The model under review builds one solid part; all positions refer to its coordinate system, in mm. A direction names the side the tool comes from. Give positions to 0.01 mm unless a question says otherwise; leave off trailing zeros. Write each loop counter-clockwise with the first axis right and the second up, starting at its lowest first coordinate (ties: lowest second). Pieces come first, ordered by that corner, then holes. Notation, with made-up numbers: M -6.75,28 L 51.25,28 A24 ccw 51.25,40 Z; hole C 32,25.25 d4. An arc over 180 degrees is marked long. Write each question's results on one line, items separated by ' | '. Start each with the question number.
from build123d import *

# Parameters (mm, degrees)
F0_R         = 4.7625
F0_R_2       = 1.5
F0_R_3       = 11.2530001
F1_DEPTH     = 3.175
F2_T1_DEPTH  = 34.0506804732
F2_T6_DEPTH  = 34.0506804732
F2_T11_DEPTH = 34.0506804732


# Not quite as in the source:
# - a fillet or chamfer that OpenCascade refuses, or shapes differently, is made with other operations: its cross-section is extruded or revolved along the edge and cut away or added


with BuildPart() as f1:
    # F0 (on Top) → F1 (new body)
    with BuildSketch(Plane.XY):
        with BuildLine():
            Line((15.875, 0), (12.7, 0))
            ThreePointArc((12.7, 0), (0, -12.7), (-12.7, 0))
            Line((-12.7, 0), (-15.875, 0))
            Line((-15.875, 0), (-15.875, -19.0989050379))
            Line((-15.875, -19.0989050379), (-7.9111435612, -40.9794207753))
            ThreePointArc((-7.9111435612, -40.9794207753), (0, -46.5188631327), (7.9111435612, -40.9794207753))
            Line((7.9111435612, -40.9794207753), (15.875, -19.0989050379))
            Line((15.875, -19.0989050379), (15.875, 0))
        make_face()
        with Locations((0, -38.1)):
            Circle(F0_R, mode=Mode.SUBTRACT)
        with BuildLine():
            ThreePointArc((-12.7, 0), (0, 12.7), (12.7, 0))
            Line((12.7, 0), (15.875, 0))
            Line((15.875, 0), (15.875, 27.2180678568))
            Line((15.875, 27.2180678568), (21.5029923, 27.2180678568))
            Line((21.5029923, 27.2180678568), (21.5029923, 70.2240524568))
            Line((21.5029923, 70.2240524568), (-21.5029923, 70.2240524568))
            Line((-21.5029923, 70.2240524568), (-21.5029923, 27.2180678568))
            Line((-21.5029923, 27.2180678568), (-15.875, 27.2180678568))
            Line((-15.875, 27.2180678568), (-15.875, 0))
            Line((-15.875, 0), (-12.7, 0))
        make_face()
        with Locations((-15.4999944, 33.2210657568)):
            Circle(F0_R_2, mode=Mode.SUBTRACT)
        with Locations((-15.4999944, 64.2210545568)):
            Circle(F0_R_2, mode=Mode.SUBTRACT)
        with Locations((15.4999944, 33.2210657568)):
            Circle(F0_R_2, mode=Mode.SUBTRACT)
        with Locations((0, 48.7210601568)):
            Circle(F0_R_3, mode=Mode.SUBTRACT)
        with Locations((15.4999944, 64.2210545568)):
            Circle(F0_R_2, mode=Mode.SUBTRACT)
    extrude(amount=F1_DEPTH)

    # F2: chamfer of 6.0030106 on 4 edges, made by hand

    # F2_s2 → F2_t1 (cut)
    with BuildSketch(Plane.XY.offset(-15.4378402366)):
        Polygon((21.5029923, 64.2210418568), (15.4999817, 70.2240524568), (21.5029923, 70.2240524568), align=None)
        Polygon((-15.4999817, 70.2240524568), (-21.5029923, 64.2210418568), (-21.5029923, 70.2240524568), align=None)
    extrude(amount=F2_T1_DEPTH, mode=Mode.SUBTRACT)


with BuildPart() as f2_tool4:
    # F2_s5 → F2_t6 (new body)
    with BuildSketch(Plane.XY.offset(-15.4378402366)):
        Polygon((15.4999817, 27.2180678568), (21.5029923, 33.2210784568), (21.5029923, 27.2180678568), align=None)
    extrude(amount=F2_T6_DEPTH)

    split(bisect_by=Plane.YZ.offset(15.875), keep=Keep.TOP)


with BuildPart() as f1_1:
    add(f1.part)

    # F2_t3: cut F2_tool4
    add(f2_tool4.part, mode=Mode.SUBTRACT)


with BuildPart() as f2_tool9:
    # F2_s10 → F2_t11 (new body)
    with BuildSketch(Plane.XY.offset(-15.4378402366)):
        Polygon((-21.5029923, 33.2210784568), (-15.4999817, 27.2180678568), (-21.5029923, 27.2180678568), align=None)
    extrude(amount=F2_T11_DEPTH)

    split(bisect_by=Plane.YZ.offset(-15.875), keep=Keep.BOTTOM)


with BuildPart() as f1_2:
    add(f1_1.part)

    # F2_t8: cut F2_tool9
    add(f2_tool9.part, mode=Mode.SUBTRACT)


solid = f1_2.part
(1) Add section C-C (z = 1.55). State the section outline as (x, y) points (1 decimal).
(2) Add section D-D (y = 57). State the section outline as (x, z) points (3 decimals), then the cut area to 3 significant figures.
(3) Add section B-B (y = 0). State the section outline as (x, z) points (3 decimals), then the cut area to 3 significant figures.
(4) Clearance check with flat-ended pins moving along their axes: P1, Ø5.5, axis at x = 0, y = -38.1, coming from the +Z side; P2, Ø1.6, axis at y = -6.5, z = 1.5, coming from the +X side (3 decimals); P3, Ø1, axis at x = -2.5, z = 1, coming from the -Y side. State where each tip first meets the part, or that it passes through.
(5) Add section A-A (x = 0). State the section outline as (y, z) points (1 decimal), then the cut area to 3 significant figures.
(6) Draft analysis for pull direction X (two halves, no side actions). For faces 1 (the flat face through (18.544, 67.181, 1.565)), 2 (the flat face through (-15.875, 5, 2)), 3 (the cylindrical face through (2.198, -42.325, 1.565)), state which applies: pulls with the +X half, pulls with the -X half, needs draft (parallel to the pull), parting line crosses it, or undercut.
(7) Machinability: for faces 4 (the flat face through (15.875, 4, 2)), 5 (the flat face through (0, 26, 3.175)), which of the approach directions +Z, -Z, +X, -X, +Y, -Y give a long, thin tool a straight path to every point of the face, cutting with its end or side? Answer none if there is none.
(8) Wall thickness on L1, parallel to Y at x = 0, z = 1.8; L2, parallel to X at y = 14, z = 0.5 (3 decimals); L3, parallel to X at y = 5, z = 1.15 (3 decimals): over which ranges is each line inside the solid? List them lowest first.
Calculated:
1) outline: M -21.5,33.2 L -15.9,27.6 L -15.9,-19.1 L -7.9,-41 A8.4 ccw 7.9,-41 L 15.9,-19.1 L 15.9,27.6 L 21.5,33.2 L 21.5,64.2 L 15.5,70.2 L -15.5,70.2 L -21.5,64.2 Z; hole C -15.5,33.2 d3; hole C -15.5,64.2 d3; hole C 0,0 d25.4; hole C 0,48.7 d22.5; hole C 0,-38.1 d9.5; hole C 15.5,33.2 d3; hole C 15.5,64.2 d3
2) outline: M -21.503,0 L -7.622,0 L -7.622,3.175 L -21.503,3.175 Z; M 7.622,0 L 21.503,0 L 21.503,3.175 L 7.622,3.175 Z | area: 88.1 mm²
3) outline: M -15.875,0 L -12.7,0 L -12.7,3.175 L -15.875,3.175 Z; M 12.7,0 L 15.875,0 L 15.875,3.175 L 12.7,3.175 Z | area: 20.2 mm²
4) P1: passes through | P2: stops at x = 15.875 | P3: stops at y = -46.28
5) outline: M -46.5,0 L -42.9,0 L -42.9,3.2 L -46.5,3.2 Z; M -33.3,0 L -12.7,0 L -12.7,3.2 L -33.3,3.2 Z; M 12.7,0 L 37.5,0 L 37.5,3.2 L 12.7,3.2 Z; M 60,0 L 70.2,0 L 70.2,3.2 L 60,3.2 Z | area: 188 mm²
6) face 1: pulls with the +X half | face 2: pulls with the -X half | face 3: undercut
7) face 4: +Z, -Z, +X, -Y | face 5: +Z, +X, -X, +Y, -Y
8) L1: y = -46.52 to -42.86, -33.34 to -12.7, 12.7 to 37.47, 59.97 to 70.22 | L2: x = -15.875 to 15.875 | L3: x = -15.875 to -11.674, 11.674 to 15.875
